```python
from build123d import *

# Parameters (mm, degrees)
CROQUIS1_R              = 39.5
CROQUIS1_R_2            = 12.5
CROQUIS1_R_3            = 2
SALIENTE_EXTRUIR1_DEPTH = 25
CROQUIS3_R              = 15
CORTAR_EXTRUIR1_DEPTH   = 12
CROQUIS5_R              = 16.857920318
SALIENTE_EXTRUIR2_DEPTH = 10
CROQUIS4_R              = 1.5
CORTAR_EXTRUIR2_DEPTH   = 10
CROQUIS6_R              = 1.5
CORTAR_EXTRUIR3_DEPTH   = 12


with BuildPart() as part:
    # Croquis1 → Saliente-Extruir1 (new body)
    with BuildSketch(Plane.XY):
        Circle(CROQUIS1_R)
        Circle(CROQUIS1_R_2, mode=Mode.SUBTRACT)
        with Locations((0, 30)):
            Circle(CROQUIS1_R_3, mode=Mode.SUBTRACT)
        with Locations((30, 0)):
            Circle(CROQUIS1_R_3, mode=Mode.SUBTRACT)
        with Locations((0, -30)):
            Circle(CROQUIS1_R_3, mode=Mode.SUBTRACT)
        with Locations((-30, 0)):
            Circle(CROQUIS1_R_3, mode=Mode.SUBTRACT)
    extrude(amount=SALIENTE_EXTRUIR1_DEPTH)

    # Croquis3 → Cortar-Extruir1 (cut)
    with BuildSketch(Plane.XY.offset(25)):
        Circle(CROQUIS3_R)
        Polygon((17.67766953, 13.435028843), (25.455844123, 21.213203436), (21.213203436, 25.455844123), (13.435028843, 17.67766953), align=None)
        Polygon((13.435028843, -17.67766953), (21.213203436, -25.455844123), (25.455844123, -21.213203436), (17.67766953, -13.435028843), align=None)
        Polygon((-17.67766953, -13.435028843), (-25.455844123, -21.213203436), (-21.213203436, -25.455844123), (-13.435028843, -17.67766953), align=None)
        Polygon((-13.435028843, 17.67766953), (-21.213203436, 25.455844123), (-25.455844123, 21.213203436), (-17.67766953, 13.435028843), align=None)
    extrude(amount=-CORTAR_EXTRUIR1_DEPTH, mode=Mode.SUBTRACT)

    # Croquis5 → Saliente-Extruir2 (add)
    with BuildSketch(Plane(origin=(0, 0, 0), x_dir=(-1, 0, 0), z_dir=(0, 0, -1))):
        Circle(CROQUIS5_R)
    extrude(amount=-SALIENTE_EXTRUIR2_DEPTH)

    # Croquis4 → Cortar-Extruir2 (cut)
    with BuildSketch(Plane(origin=(0, 0, 0), x_dir=(-1, 0, 0), z_dir=(0, 0, -1))):
        with Locations((-12.727922061, -6.363961031)):
            Circle(CROQUIS4_R)
        with Locations((-6.363961031, -12.727922061)):
            Circle(CROQUIS4_R)
        with Locations((21.920310217, 28.284271247)):
            Circle(CROQUIS4_R)
        with Locations((28.284271247, 21.920310217)):
            Circle(CROQUIS4_R)
        Polygon((30, -3.5), (33.031088913, -1.75), (33.031088913, 1.75), (30, 3.5), (26.968911087, 1.75), (26.968911087, -1.75), align=None)
        Polygon((3.5, 30), (1.75, 33.031088913), (-1.75, 33.031088913), (-3.5, 30), (-1.75, 26.968911087), (1.75, 26.968911087), align=None)
        Polygon((-3.5, -30), (-1.75, -33.031088913), (1.75, -33.031088913), (3.5, -30), (1.75, -26.968911087), (-1.75, -26.968911087), align=None)
        Polygon((-30, 3.5), (-33.031088913, 1.75), (-33.031088913, -1.75), (-30, -3.5), (-26.968911087, -1.75), (-26.968911087, 1.75), align=None)
        Polygon((0.353553391, -13.788582233), (29.344931419, 15.202795796), (15.202795796, 29.344931419), (-13.788582233, 0.353553391), align=None)
    extrude(amount=-CORTAR_EXTRUIR2_DEPTH, mode=Mode.SUBTRACT)

    # Croquis6 → Cortar-Extruir3 (cut)
    with BuildSketch(Plane(origin=(0, 0, 0), x_dir=(-1, 0, 0), z_dir=(0, 0, -1))):
        with Locations((-12.727922061, -6.363961031)):
            Circle(CROQUIS6_R)
        with Locations((-6.363961031, -12.727922061)):
            Circle(CROQUIS6_R)
        with Locations((21.920310217, 28.284271247)):
            Circle(CROQUIS6_R)
        with Locations((28.284271247, 21.920310217)):
            Circle(CROQUIS6_R)
    extrude(amount=-CORTAR_EXTRUIR3_DEPTH, mode=Mode.SUBTRACT)


solid = part.part
```
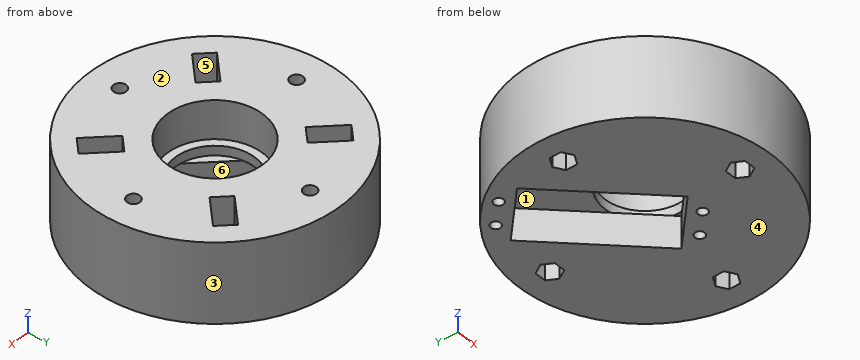
Could you check a few things on this model? Use its own coordinates, in mm. Face numbers are marked on the shaded views. A direction names the side the tool comes from. Coordinates: 2 decimals unless noted, no trailing zeros. Write each loop counter-clockwise with the first axis right and the second up, starting at its lowest first coordinate (ties: lowest second). Pieces come first, ordered by that corner, then holes. Notation, with made-up numbers: (-36.5, 72) - (-9.5, 72) arc R6 ccw to (-9.5, 79) - close; hole circle Ø11 at (52, 70). An arc over 180 degrees is marked (long way). Use a Markdown table: item, result.
Q1. Please list where these lines run through material, in increasing order: L1, parallel to Y at x = 0, z = 12.4; L2, parallel to Y at x = 0, z = 18; L3, parallel to Y at x = 7, z = 5.5.
Geometry check:
| item | result |
|---|---|
| L1 | y = -39.5 to -32, -28 to -12.5, 12.5 to 28, 32 to 39.5 |
| L2 | y = -39.5 to -32, -28 to -15, 15 to 28, 32 to 39.5 |
| L3 | y = -38.87 to -14.09, -11.37 to -6.44, 7.14 to 38.87 |
Q2. Imagine slicing it at D-D (y = -34). List the corners of the cut face in (x, z) for me, and give its area (3 significant figures).
Geometry check:
| item | result |
|---|---|
| outline | (-20.11, 0) - (20.11, 0) - (20.11, 25) - (-20.11, 25) - close |
| area | 1,010 mm2 |
Q3. Imagine slicing it at A-A (z = 14.75). Count the separate pieces of the cut face and the enclosed holes in it, and give its area (3 significant figures).
Geometry check:
| item | result |
|---|---|
| separate pieces | 1 |
| enclosed holes | 9 |
| area | 3,880 mm2 |
Q4. Which directions (+Z, -Z, +X, -X, +Y, -Y) give clear straight access to the entire face, cutting with the end or side of a thin tool? Please do the marked faces 4, 5 and 6.
Geometry check:
| item | result |
|---|---|
| face 4 | -Z, +X, -X, +Y, -Y |
| face 5 | +Z |
| face 6 | -Z |
Q5. Imagine slicing it at B-B (y = 31). List the corners of the cut face in (x, z) for me, and give its area (3 significant figures).
Geometry check:
| item | result |
|---|---|
| outline | (-24.48, 0) - (-2.92, 0) - (-2.92, 10) - (-1.73, 10) - (-1.73, 25) - (-24.48, 25) - close; (1.73, 10) - (2.92, 10) - (2.92, 0) - (24.48, 0) - (24.48, 25) - (1.73, 25) - close |
| area | 1,110 mm2 |
Q6. I'm going to push flat-ended pins straight in: pin 1 Ø9.5 at (x, y) = (-18.5, 19) entering from -Z; pin 2 Ø0.9 at (x, y) = (-22, 27.5) entering from -Z; pin 3 Ø1 at (x, z) = (0, 5) entering from -Y. Where does each tip first touch, or does it pass through?
Geometry check:
| item | result |
|---|---|
| pin 1 | stops at z = 10 |
| pin 2 | stops at z = 12 |
| pin 3 | stops at y = -39.5 |
Q7. Thinking about a two-plate mould opening in Y: for the marked faces 1, 2 and 3, which applies, +Y half, -Y half, draft (parallel to the pull), parting line (faces both ways), or undercut?
Geometry check:
| item | result |
|---|---|
| face 1 | undercut |
| face 2 | draft |
| face 3 | parting line |
